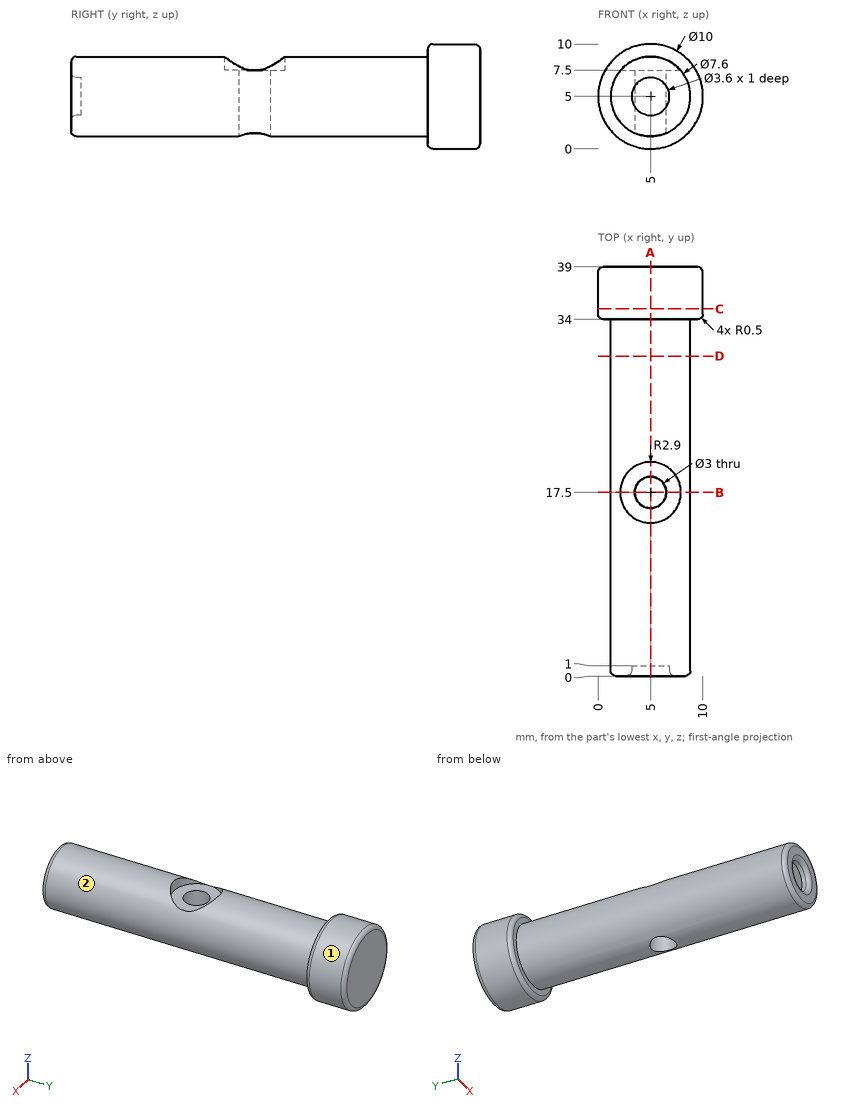
Study the drawing (mm; zero at the part's minimum x, y, z) and answer. A direction names the side the tool comes from. Give positions to 0.01 mm unless a question says otherwise; leave off trailing zeros. Loops run counter-clockwise (first coordinate to the right, second up) from the corner with the lowest first, then second, coordinate; pieces in that order, holes last. Notation, with made-up numbers: (18.25, 89.5) -> (65.25, 89.5) arc R23 cw to (65.25, 107.5) -> close; hole circle Ø6 at (-26, 36). An arc over 180 degrees is marked (long way). Write item = value, one per line. Start each with the question number.
(1) Which of the six approach directions +Z, -Z, +X, -X, +Y, -Y give full straight-line access (tool end or side, diameter ignored) to the marked faces 1 and 2?
(2) Find the intervals of material crossed by probe 1 along Z at (x, y) = (5, 0.65); probe 2 along Y at (x, z) = (5, 6); probe 3 along Y at (x, z) = (3, 4), in increasing order. Write a range as from..to.
(3) Find section D-D on y = 30.5. Give the vertices of the cut face in (x, z).
(4) Find section C-C on y = 35. Give the vertices of the cut face in (x, z).
(5) Find section B-B on y = 17.5. Give the vertices of the cut face in (x, z), and give its area (3 significant figures).
(6) Given pin 1 Ø4.5 at (x, y) = (6, 19) entering from +Z; pin 2 Ø1.5 at (y, z) = (20, 2.5) entering from -X; pin 3 Ø4.5 at (x, z) = (5, 5) entering from -Y, each flat-ended and moving along its own axis, determine where each tip first touches the part or whether it passes through.
(7) Find section A-A on x = 5. Give the vertices of the cut face in (y, z).
From the geometry:
q1.face_1 = +Y, -Y
q1.face_2 = -Y
q2.probe_1 = 1.2..3.2, 6.8..8.8
q2.probe_2 = 1..16, 19..39
q2.probe_3 = 0..39
q3.outline = circle Ø7.6 at (5, 5)
q4.outline = circle Ø10 at (5, 5)
q5.outline = (2.14, 7.5) arc R3.8 ccw to (3.5, 1.51) -> (3.5, 7.5) -> close; (6.5, 1.51) arc R3.8 ccw to (7.86, 7.5) -> (6.5, 7.5) -> close
q5.area = 21.6 mm^2
q6.pin_1 = 8.8
q6.pin_2 = 1.63
q6.pin_3 = 0
q7.outline = (0, 1.7) arc R0.5 ccw to (0.5, 1.2) -> (16, 1.2) -> (16, 7.5) -> (14.6, 7.5) -> (14.6, 8.8) -> (0.5, 8.8) arc R0.5 ccw to (0, 8.3) -> (0, 7.3) arc R0.5 ccw to (0.5, 6.8) -> (1, 6.8) -> (1, 3.2) -> (0.5, 3.2) arc R0.5 ccw to (0, 2.7) -> close; (19, 1.2) -> (34, 1.2) -> (34, 0.5) arc R0.5 ccw to (34.5, 0) -> (38.5, 0) arc R0.5 ccw to (39, 0.5) -> (39, 9.5) arc R0.5 ccw to (38.5, 10) -> (34.5, 10) arc R0.5 ccw to (34, 9.5) -> (34, 8.8) -> (20.4, 8.8) -> (20.4, 7.5) -> (19, 7.5) -> close
